from build123d import *

# Parameters (mm, degrees)
F1_DEPTH = 15.494


# Not quite as in the source:
# - the program builds the solid bodies; features that only make, move or delete a surface that nothing else refers to are left out


with BuildPart() as f1:
    # F0 (on Front) → F1 (new body)
    with BuildSketch(Plane.XZ):
        with BuildLine():
            Line((1.9883703665, 34.5010177122), (8.7319990578, 68.2588214835))
            ThreePointArc((8.7319990578, 68.2588214835), (5.9467168888, 68.5576478309), (3.1515805748, 68.742869141))
            Line((3.1515805748, 68.742869141), (-3.7173636083, 34.3577509115))
            ThreePointArc((-3.7173636083, 34.3577509115), (-0.867459366, 34.5473783975), (1.9883703665, 34.5010177122))
        make_face()
        with BuildLine():
            ThreePointArc((3.1515805748, 68.742869141), (-49.7613844804, -47.5322956783), (68.8150747864, 0))
            ThreePointArc((68.8150747864, 0), (51.6546594513, 45.4676882503), (8.7319990578, 68.2588214835))
            Line((8.7319990578, 68.2588214835), (1.9883703665, 34.5010177122))
            ThreePointArc((1.9883703665, 34.5010177122), (25.1295490861, 23.7229762598), (34.5582673161, 0))
            ThreePointArc((34.5582673161, 0), (-23.0847156643, -25.717109919), (-3.7173636083, 34.3577509115))
            Line((-3.7173636083, 34.3577509115), (3.1515805748, 68.742869141))
        make_face()
    extrude(amount=F1_DEPTH)


solid = f1.part
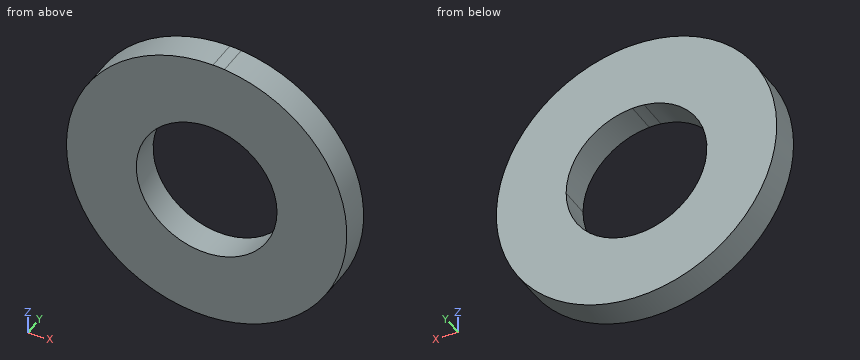
For this review, take the finished solid that the model builds, in its own axes (mm). Round coordinates to 2 decimals unless told otherwise and drop trailing zeros. Loops run counter-clockwise (first coordinate to the right, second up) from the corner with the lowest first, then second, coordinate; pieces in that order, holes last. Notation, with made-up numbers: (-12.75, 46) - (36.25, 46) arc R17 ccw to (36.25, 68) - close; hole circle Ø1 at (20.5, 9.5). An arc over 180 degrees is marked (long way). One line per item, written item: value. Start each with the question number.
Item 1: Take a section at A-A (x = 0). Give the boundary of the cut face in (y, z), plus the area to 3 significant figures.
Item 2: Take a section at D-D (z = 58). Give the boundary of the cut face in (x, y), plus the area to 3 significant figures.
Item 3: Take a section at C-C (y = -10.25). Give the boundary of the cut face in (x, z), plus the area to 3 significant figures.
Item 4: For L1, parallel to Z at x = 0, y = -8.5; L2, parallel to X at y = -8.75, z = 11, list the stretches that pass through material, from the lowest coordinate up.
Item 5: Take a section at B-B (z = 31.5). Give the boundary of the cut face in (x, y), plus the area to 3 significant figures.
Item 6: Clearance check with flat-ended pins moving along their axes: pin 1 Ø2 at (x, y) = (10.5, -5) entering from -Z; pin 2 Ø6 at (y, z) = (-5, 50.5) entering from +X; pin 3 Ø1.5 at (x, y) = (3.5, -4) entering from +Z. State where each tip first meets the part, or that it passes through.
Answer below:
1. outline: (-15.49, -68.82) - (0, -68.82) - (0, -34.56) - (-15.49, -34.56) - close; (-15.49, 34.56) - (0, 34.56) - (0, 68.82) - (-15.49, 68.82) - close
1. area: 1,060 mm2
2. outline: (-37.03, -15.49) - (37.03, -15.49) - (37.03, 0) - (-37.03, 0) - close
2. area: 1,150 mm2
3. outline: circle Ø137.63 at (0, 0); hole circle Ø69.12 at (0, 0)
3. area: 11,100 mm2
4. L1: z = -68.82 to -34.56, 34.56 to 68.82
4. L2: x = -67.93 to -32.76, 32.76 to 67.93
5. outline: (-61.18, -15.49) - (-14.21, -15.49) - (-14.21, 0) - (-61.18, 0) - close; (14.21, -15.49) - (61.18, -15.49) - (61.18, 0) - (14.21, 0) - close
5. area: 1,460 mm2
6. pin 1: stops at z = -68.16
6. pin 2: stops at x = 49.79
6. pin 3: stops at z = 68.76
